```python
from build123d import *

# Parameters (mm, degrees)
SKETCH1_W           = 40.5
SKETCH1_H           = 56
BOSS_EXTRUDE1_DEPTH = 3
FILLET1_R           = 3
SHELL1_T            = -1.5
SKETCH2_W           = 5
SKETCH2_H           = 3
BOSS_EXTRUDE2_DEPTH = 1.5
SKETCH3_W           = 1.9
SKETCH3_H           = 5
BOSS_EXTRUDE3_DEPTH = 3
SKETCH8_W           = 5
SKETCH8_H           = 3
BOSS_EXTRUDE5_DEPTH = 1.5
SKETCH9_W           = 5
SKETCH9_H           = 1.9
BOSS_EXTRUDE6_DEPTH = 3


with BuildPart() as part:
    # Sketch1 → Boss-Extrude1 (new body)
    with BuildSketch(Plane(origin=(0, 0, 0), x_dir=(1, 0, 0), z_dir=(0, 1, 0))):
        with Locations((20.25, 28)):
            Rectangle(SKETCH1_W, SKETCH1_H)
    extrude(amount=BOSS_EXTRUDE1_DEPTH)

    # Fillet1
    fillet1_edges = [part.edges().sort_by_distance(p)[0] for p in [
        (0, 1.5, -56),
        (40.5, 1.5, -56),
        (40.5, 1.5, 0),
        (0, 1.5, 0),
    ]]
    fillet(fillet1_edges, radius=FILLET1_R)

    # Shell1
    shell1_openings = [part.faces().sort_by_distance(p)[0] for p in [
        (20.25, 3, -28),
    ]]
    offset(amount=SHELL1_T, openings=shell1_openings, kind=Kind.INTERSECTION)

    # Sketch2 → Boss-Extrude2 (add)
    with BuildSketch(Plane.ZY):
        with Locations((-28.5, 1.5)):
            Rectangle(SKETCH2_W, SKETCH2_H)
    boss_extrude2 = extrude(amount=BOSS_EXTRUDE2_DEPTH)

    # Sketch3 → Boss-Extrude3 (add)
    with BuildSketch(Plane(origin=(0, 3, 0), x_dir=(1, 0, 0), z_dir=(0, 1, 0))):
        with Locations((-0.55, 28.5)):
            Rectangle(SKETCH3_W, SKETCH3_H)
    boss_extrude3 = extrude(amount=BOSS_EXTRUDE3_DEPTH)

    # Sketch8 → Boss-Extrude5 (add)
    with BuildSketch(Plane.XY):
        with Locations((19.75, 1.5)):
            Rectangle(SKETCH8_W, SKETCH8_H)
    boss_extrude5 = extrude(amount=BOSS_EXTRUDE5_DEPTH)

    # Sketch9 → Boss-Extrude6 (add)
    with BuildSketch(Plane(origin=(0, 3, 0), x_dir=(1, 0, 0), z_dir=(0, 1, 0))):
        with Locations((19.75, -0.55)):
            Rectangle(SKETCH9_W, SKETCH9_H)
    boss_extrude6 = extrude(amount=BOSS_EXTRUDE6_DEPTH)

    # Mirror3: Boss-Extrude2, Boss-Extrude3 across plane
    add(boss_extrude2.mirror(Plane(origin=(20.25, 0, 0), x_dir=(0, 0, 1), z_dir=(1, 0, 0))))
    add(boss_extrude3.mirror(Plane(origin=(20.25, 0, 0), x_dir=(0, 0, 1), z_dir=(1, 0, 0))))

    # Mirror4: Boss-Extrude5, Boss-Extrude6 across plane
    add(boss_extrude5.mirror(Plane(origin=(0, 0, -28), x_dir=(1, 0, 0), z_dir=(0, 0, -1))))
    add(boss_extrude6.mirror(Plane(origin=(0, 0, -28), x_dir=(1, 0, 0), z_dir=(0, 0, -1))))


solid = part.part
```
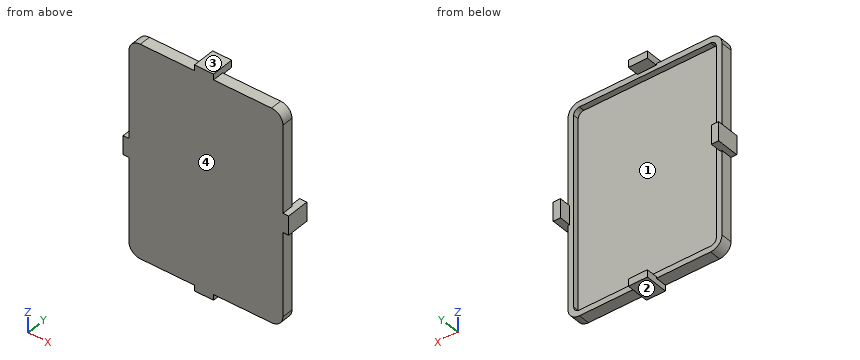
Input: part model. Units: mm. Frame: model coordinates. Face numbers are marked on the shaded views. Round coordinates to 2 decimals unless told otherwise and drop trailing zeros. Loops run counter-clockwise (first coordinate to the right, second up) from the corner with the lowest first, then second, coordinate; pieces in that order, holes last. Notation, with made-up numbers: (51, 2.25) - (70, 2.25) arc R11 ccw to (70, 23.25) - close; hole circle Ø3 at (31, 86). An arc over 180 degrees is marked (long way). One line per item, written item: value. Start each with the question number.
(1) Section B-B, the plane z = -9. Return loops of the section in (x, y), plus the area to 4 significant figures.
(2) Ray query, line 1 (Z direction, x = 19, y = 5.7); line 2 (X direction, y = 2.6, z = -22.5); line 3 (Z direction, x = 17.5, y = 1.6). Return the intervals inside material, ascending. Write a range as [from, to].
(3) Section C-C, the plane x = 34. Return loops of the section in (y, z), plus the area to 3 significant figures.
(4) Draft query along Z for the marked faces 1, 2, 3 and 4. Return one class per face: +Z half, -Z half, draft (parallel to the pull), parting line (faces both ways), or undercut.
(5) Contact query for flat-ended pins moving along their axis: P1, Ø1, axis at x = 29.5, y = 1.5, coming from the +Z side; P2, Ø1.6, axis at y = 2.5, z = -40, coming from the -X side; P3, Ø1.5, axis at y = 1, z = -42, coming from the +X side. Output: stop coordinate, or through.
(6) Section A-A, the plane y = 4.9. Return loops of the section in (x, z).
Results below:
1. outline: (0, 0) - (40.5, 0) - (40.5, 3) - (39, 3) - (39, 1.5) - (1.5, 1.5) - (1.5, 3) - (0, 3) - close
1. area: 65.25 mm^2
2. line 1: [-57.5, -55.6], [-0.4, 1.5]
2. line 2: [0, 1.5], [39, 40.5]
2. line 3: [-57.5, -54.5], [-1.5, 1.5]
3. outline: (0, -56) - (3, -56) - (3, -54.5) - (1.5, -54.5) - (1.5, -1.5) - (3, -1.5) - (3, 0) - (0, 0) - close
3. area: 88.5 mm^2
4. face 1: undercut
4. face 2: -Z half
4. face 3: +Z half
4. face 4: draft
5. P1: z = 0
5. P2: x = 0
5. P3: x = 40.5
6. outline: (-1.5, -31) - (0.4, -31) - (0.4, -26) - (-1.5, -26) - close; (17.25, -57.5) - (22.25, -57.5) - (22.25, -55.6) - (17.25, -55.6) - close; (17.25, -0.4) - (22.25, -0.4) - (22.25, 1.5) - (17.25, 1.5) - close; (40.1, -31) - (42, -31) - (42, -26) - (40.1, -26) - close
